The model under review builds one solid part; all positions refer to its coordinate system, in mm. A direction names the side the tool comes from. Coordinates: 2 decimals unless noted, no trailing zeros. Write each loop counter-clockwise with the first axis right and the second up, starting at its lowest first coordinate (ties: lowest second). Pieces come first, ordered by that corner, then holes.
1) Add section B-B, the plane z = -28. State the section outline as (x, y) points.
2) Add section D-D, the plane x = -38. State the section outline as (y, z) points, then the cut area to 3 significant figures.
3) Machinability: for faces 1 (the flat face through (-2, 0, 2)), 2 (the cylindrical face through (0.75, -83.83, -0.58)), which of the approach directions +Z, -Z, +X, -X, +Y, -Y give a long, thin tool a straight path to every point of the face, cutting with its end or side? Answer none if there is none.
4) Add section A-A, the plane x = 63. State the section outline as (y, z) points, then the cut area to 3 significant figures.
5) For P1, Ø4, axis at x = -34, z = 32.5, coming from the -Y side; P2, Ø12, axis at y = -73, z = 40, coming from the +X side, all flat-tipped, find the tip position at first contact; note any pin that passes through.
6) For line 1 (Y direction, x = 57, z = 17); line 2 (Z direction, x = -15, y = -67.5); line 3 (Z direction, x = 59.5, y = -78), list the stretches that pass through material, from the lowest coordinate up.
from build123d import *

# Parameters (mm, degrees)
F0_W     = 151.190631
F0_H     = 153.706558
F1_DEPTH = 65.923417
F3_DEPTH = 36.313294


with BuildPart() as f1:
    # F0 (on Front) → F1 (new body)
    with BuildSketch(Plane.XZ):
        with Locations((-0.911687, 0.695508)):
            Rectangle(F0_W, F0_H)
    extrude(amount=F1_DEPTH)

    # F2 (on face) → F3 (join)
    with BuildSketch(Plane.XZ.offset(65.923417)):
        with BuildLine():
            Line((-76.507002, -76.157771), (74.683629, -76.157771))
            ThreePointArc((74.683629, -76.157771), (-0.911687, -0.562456), (-76.507002, -76.157771))
        make_face()
    extrude(amount=F3_DEPTH)


solid = f1.part
Geometry results:
1. outline: (-76.51, -65.92) - (-59.18, -65.92) - (-59.18, -102.24) - (57.36, -102.24) - (57.36, -65.92) - (74.68, -65.92) - (74.68, 0) - (-76.51, 0) - close
2. outline: (-102.24, -76.16) - (0, -76.16) - (0, 77.55) - (-65.92, 77.55) - (-65.92, -10.29) - (-102.24, -10.29) - close
2. area: 12,500 mm2
3. face 1: +Z, -Z, +X, -X, +Y
3. face 2: +Z, -Y
4. outline: (-102.24, -76.16) - (0, -76.16) - (0, 77.55) - (-65.92, 77.55) - (-65.92, -35.79) - (-102.24, -35.79) - close
4. area: 11,600 mm2
5. P1: stops at y = -65.92
5. P2: passes through
6. line 1: y = -65.92 to 0
6. line 2: z = -76.16 to -1.89
6. line 3: z = -76.16 to -30.71
